Check sheet for the modelled part. Datum: model origin and axes. Units: mm. Face numbers are marked on the shaded views. A direction names the side the tool comes from. Give positions to 0.01 mm unless a question says otherwise; leave off trailing zeros. Write each loop counter-clockwise with the first axis right and the second up, starting at its lowest first coordinate (ties: lowest second). Pieces come first, ordered by that corner, then holes. Notation, with made-up numbers: (84.25, 68.25) -> (137.25, 68.25) arc R18 cw to (137.25, 97.25) -> close; hole circle Ø6 at (85.25, -12.75). An arc over 180 degrees is marked (long way). Use a Markdown table: item, result. Add a question column.
1. Scan lines: probe 1 along Y at (x, z) = (37.5, 1.75); probe 2 along Z at (x, y) = (4.5, 14.75); probe 3 along X at (y, z) = (2.75, 16.5). Record each from-to range of solid material in increasing order. Write a range as [from, to].
2. Cross-section at B-B (y = 10). Enter the section's corners in (x, z), then the cut area to 3 significant figures.
3. Cross-section at A-A (z = 18.25). Enter the section's corners in (x, y) (3 decimals), then the cut area to 3 significant figures.
4. Set-up check for the marked faces 1, 2, 3, 4 and 5: record each of +Z, -Z, +X, -X, +Y, -Y from which the full face is reachable in a straight line by a thin tool's end or side.
5. Release check for a two-part mould opening along X. For the marked faces 6, 7 and 8 record: released by +X, released by -X, zero draft, split by the parting line, or undercut.
6. Gauge pin test, flat ends, axial feed: P1, Ø2, axis at x = 41, z = 17.5, coming from the -Y side; P2, Ø2, axis at x = 19, y = 16.5, coming from the +Z side; P3, Ø6, axis at y = 18, z = 7, coming from the -X side. Record the tip position at first contact, or that the pin passes through.
7. Cross-section at D-D (x = 36). Enter the section's corners in (y, z).
8. Cross-section at C-C (z = 5). Enter the section's corners in (x, y) (3 decimals).
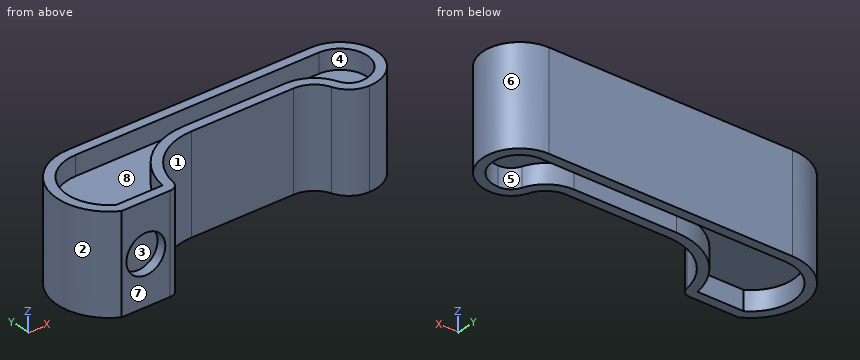
from build123d import *

# Parameters (mm, degrees)
BOSS_EXTRUDE1_DEPTH = 20
CUT_EXTRUDE1_DEPTH  = 4
SKETCH4_R           = 4
CUT_EXTRUDE2_DEPTH  = 2


with BuildPart() as part:
    # Sketch1 → Boss-Extrude1 (new body)
    with BuildSketch(Plane.XY):
        with BuildLine():
            Line((0, 0), (10, 0))
            ThreePointArc((10, 0), (11.31707778, 0.487218781), (12, 1.714285714))
            ThreePointArc((12, 1.714285714), (16.097533322, 9.076687314), (24, 12))
            Line((24, 12), (45, 12))
            ThreePointArc((45, 12), (48.051638904, 11.038055577), (50, 8.5))
            ThreePointArc((50, 8.5), (51.948361096, 5.961944423), (55, 5))
            ThreePointArc((55, 5), (62.5, 12.5), (55, 20))
            Line((55, 20), (5, 20))
            ThreePointArc((5, 20), (-5.307764064, 11.951941016), (0, 0))
        make_face()
    extrude(amount=BOSS_EXTRUDE1_DEPTH)

    # Sketch3 → Cut-Extrude1 (cut)
    with BuildSketch(Plane.XY.offset(20)):
        with BuildLine():
            Line((24, 14), (45, 14))
            ThreePointArc((45, 14), (49.198563593, 12.676519418), (51.879194631, 9.184563758))
            ThreePointArc((51.879194631, 9.184563758), (53.095285785, 7.600408264), (55, 7))
            ThreePointArc((55, 7), (60.5, 12.5), (55, 18))
            Line((55, 18), (5, 18))
            ThreePointArc((5, 18), (-3.306623863, 11.696771953), (0.527864045, 2))
            Line((0.527864045, 2), (10, 2))
            ThreePointArc((10, 2), (10.015495033, 2.005731986), (10.023529412, 2.020168067))
            ThreePointArc((10.023529412, 2.020168067), (14.795950575, 10.595200519), (24, 14))
        make_face()
    cut_extrude1 = extrude(amount=-CUT_EXTRUDE1_DEPTH, mode=Mode.SUBTRACT)

    # Mirror1: Cut-Extrude1 across plane
    add(cut_extrude1.mirror(Plane.XY.offset(10)), mode=Mode.SUBTRACT)

    # Sketch4 → Cut-Extrude2 (cut)
    with BuildSketch(Plane(origin=(0, 0, 0), x_dir=(-1, 0, 0), z_dir=(0, -1, 0))):
        with Locations(Location((-5, -10, 0), (0, 0, 90))):
            Circle(SKETCH4_R)
    extrude(amount=-CUT_EXTRUDE2_DEPTH, mode=Mode.SUBTRACT)


solid = part.part
Worked answers:
| question | item | result |
|---|---|---|
| 1 | probe 1 | y = [12, 14], [18, 20] |
| 1 | probe 2 | z = [4, 16] |
| 1 | probe 3 | x = [-3.31, -0.52], [10.16, 12.21] |
| 2 | outline | (-5.61, 0) -> (-3.6, 0) -> (-3.6, 4) -> (14.14, 4) -> (14.14, 0) -> (17.32, 0) -> (17.32, 20) -> (14.14, 20) -> (14.14, 16) -> (-3.6, 16) -> (-3.6, 20) -> (-5.61, 20) -> close; (49.16, 0) -> (51.52, 0) -> (51.52, 4) -> (59.9, 4) -> (59.9, 0) -> (62.07, 0) -> (62.07, 20) -> (59.9, 20) -> (59.9, 16) -> (51.52, 16) -> (51.52, 20) -> (49.16, 20) -> close |
| 2 | area | 508 mm² |
| 3 | outline | (0, 0) -> (10, 0) arc R2.024 ccw to (12, 1.714) arc R12.143 cw to (24, 12) -> (45, 12) arc R5.321 cw to (50, 8.5) arc R5.321 ccw to (55, 5) arc R7.5 ccw to (55, 20) -> (5, 20) arc R10.625 ccw to start; hole (0.528, 2) -> (10, 2) arc R0.024 ccw to (10.024, 2.02) arc R14.143 cw to (24, 14) -> (45, 14) arc R7.321 cw to (51.879, 9.185) arc R3.321 ccw to (55, 7) arc R5.5 ccw to (55, 18) -> (5, 18) arc R8.625 ccw to start |
| 3 | area | 319 mm² |
| 4 | face 1 | +Z, -Z, -Y |
| 4 | face 2 | +Z, -Z, -X |
| 4 | face 3 | -Y |
| 4 | face 4 | +Z |
| 4 | face 5 | -Z |
| 5 | face 6 | released by +X |
| 5 | face 7 | zero draft |
| 5 | face 8 | undercut |
| 6 | P1 | stops at y = 12 |
| 6 | P2 | stops at z = 16 |
| 6 | P3 | stops at x = -4.01 |
| 7 | outline | (12, 0) -> (14, 0) -> (14, 4) -> (18, 4) -> (18, 0) -> (20, 0) -> (20, 20) -> (18, 20) -> (18, 16) -> (14, 16) -> (14, 20) -> (12, 20) -> close |
| 8 | outline | (0, 0) -> (10, 0) arc R2.024 ccw to (12, 1.714) arc R12.143 cw to (24, 12) -> (45, 12) arc R5.321 cw to (50, 8.5) arc R5.321 ccw to (55, 5) arc R7.5 ccw to (55, 20) -> (5, 20) arc R10.625 ccw to start |
